For this review, take the finished solid that the model builds, in its own axes (mm). Face numbers are marked on the shaded views. A direction names the side the tool comes from. Round coordinates to 2 decimals unless told otherwise and drop trailing zeros. Order: outer loops, then holes, each group sorted by start corner. A loop starts at its lowest first (then second) coordinate and runs counter-clockwise, first axis right, second up. Notation, with made-up numbers: (12, -29) -> (28, -29) arc R4 ccw to (28, -23) -> close; hole circle Ø6 at (80.5, -19). An arc over 180 degrees is marked (long way). Answer in a Markdown table with one row per item.
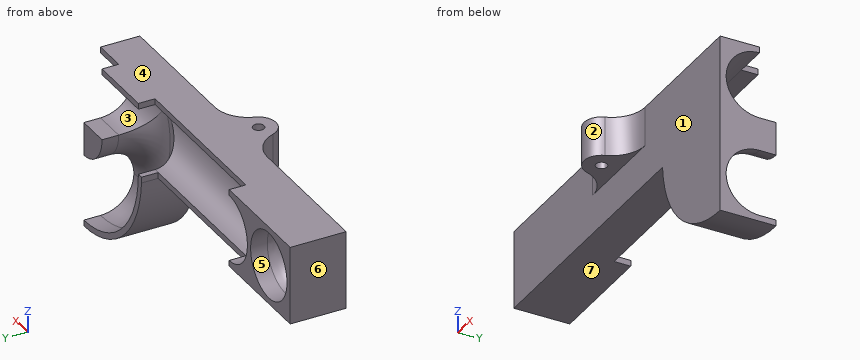
Autodesk Inventor part; units mm, degrees
ref_plane "YZ Plane" through (0, 0, 0) normal (1, 0, 0) x (0, 1, 0)
ref_plane "XZ Plane" through (0, 0, 0) normal (0, 1, 0) x (-1, 0, 0)
ref_plane "XY Plane" through (0, 0, 0) normal (0, 0, 1) x (1, 0, 0)
sketch "Esboço1" plane through (0, 0, 0) normal (0, 1, 0) x (-1, 0, 0)
  arc A0 (-102.2, -28.6) -> (-93.2, -19.6) centre (-102.2, -19.6) ccw
  arc A1 (-102.2, -46.6) -> (-75.2, -19.6) centre (-102.2, -19.6) ccw
  line L0 (-75.2, -19.6) -> (-30.2, -19.6)
  line L1 (-93.2, -19.6) -> (-102.2, -19.6)
  line L2 (-102.2, -19.6) -> (-102.2, -1.6)
  line L3 (-102.2, -1.6) -> (-93.2, -1.6)
  line L4 (-93.2, -1.6) -> (-75.2, -1.6)
  line L5 (-75.2, -1.6) -> (-30.2, -1.6)
  arc A2 (-30.2, -19.6) -> (-30.2, -1.6) centre (-30.2, -10.6) ccw
  line L6 (-102.2, -28.6) -> (-102.2, -46.6)
  arc A3 (-102.2, -48.2) -> (-73.6448, -21.2) centre (-102.2, -19.6) ccw
  arc A4 (-102.2, -27) -> (-94.975, -21.2) centre (-102.2, -19.6) ccw
  line L7 (-94.975, -21.2) -> (-102.2, -21.2)
  line L8 (-102.2, 0) -> (-93.2, 0)
  line L9 (-93.2, 0) -> (-75.2, 0)
  line L10 (-75.2, 0) -> (0, 0)
  line L11 (0, -21.2) -> (-73.6448, -21.2)
  line L12 (-73.6448, -21.2) -> (-73.6448, -19.6)
  line L13 (-102.2, -46.6) -> (-102.2, -48.2)
  line L14 (-102.2, -28.6) -> (-102.2, -27)
  line L15 (-102.2, -21.2) -> (-102.2, -19.6)
  line L16 (-102.2, -1.6) -> (-102.2, 0)
  line L17 (-94.975, -21.2) -> (-94.975, -19.6)
  line L18 (-93.2, -1.6) -> (-93.2, 0)
  line L19 (-75.2, -1.6) -> (-75.2, 0)
  line L20 (0, -21.2) -> (0, 0)
  circle A5 centre (-10.6, -10.6) radius 9
  line L21 (-30.2, -21.2) -> (-30.2, -19.6)
  line L22 (-30.2, -1.6) -> (-30.2, 0)
  line L23 (-102.2, -21.2) -> (-102.2, -27)
  point P0 (-21.2, -10.6)
  point P1 (-73.6448, -21.2)
  point P2 (-30.2, -1.6)
  point P3 (-30.2, -19.6)
  dimension "d20" = 18
  dimension "d21" = 18
  dimension "d22" = 54
  dimension "d23" = 1.6
  dimension "d30" = 1.6
  dimension "d31" = 1.6
  dimension "d32" = 1.6
  dimension "d33" = 9
  dimension "d35" = 18
  dimension "d38" = 1.6
  dimension "d44" = 1.6
  dimension "d45" = 1.6
extrude "Margem externa" add sketch "Esboço1" against normal blind 1.6 contours L14 A4 L17 L1 A0 | A0 L1 L2 L3 L4 L5 A2 L0 A1 L6 | A1 L0 L12 A3 L13 | L23 L7 A4 | L17 L7 L15 L1 | L0 L21 L11 L12 | L16 L8 L18 L3 | A2 L22 L10 L20 L11 L21 | L18 L9 L19 L4 | L5 L19 L10 L22 | A5
extrude "Proteção alta" add sketch "Esboço1" along normal blind 13.5 contours L14 A4 L17 L1 A0 | A1 L0 L12 A3 L13 | L23 L7 A4 | L17 L7 L15 L1 | A2 L22 L10 L20 L11 L21 | L18 L9 L19 L4
extrude "Proteção baixa" add sketch "Esboço1" along normal blind 9 contours L14 A4 L17 L1 A0 | A1 L0 L12 A3 L13 | L17 L7 L15 L1 | L0 L21 L11 L12 | L16 L8 L18 L3 | A2 L22 L10 L20 L11 L21 | L18 L9 L19 L4 | L5 L19 L10 L22
fillet "Arredondamento3" radius 9 7 edges at (19.6, 0, -10.6) (66.2, 0, -1.6) (52.7, 0, -19.6) (21.2, 0, -10.6) (83.1081, 0, -38.6919) (97.7, 0, -19.6) (95.836, 0, -25.964)
sketch "Esboço2" plane through (0, -1.6, 0) normal (0, -1, 0) x (1, 0, 0)
  line L0 (59.514, 0) -> (44.514, 0)
  line L1 (44.514, 0) -> (44.514, -10.6)
  line L2 (44.514, -10.6) -> (59.514, -10.6)
  line L3 (59.514, -10.6) -> (59.514, 0)
  line L4 (0, 0) -> (0, -21.2)
  point P0 (52.014, -10.6)
  point P1 (0, -10.6)
  point P2 (52.014, 0)
  dimension "d47" = 52.014
  dimension "d48" = 15
extrude "Extrusão5" add sketch "Esboço2" along normal blind 9.4
sketch "Esboço3" plane through (59.514, -1.6, -10.6) normal (0, 0, -1) x (-1, 0, 0)
  circle A0 centre (7.5, -4.7) radius 1.5
  line L0 (15, -9.4) -> (0, -9.4)
  line L1 (15, 0) -> (15, -9.4)
  line L2 (59.514, 0) -> (-14.1308, 0)
  line L3 (12.2, 0) -> (15, 0)
  line L4 (15, 0) -> (15, -9.4)
  line L5 (15.1598, -9.4) -> (0, -9.4)
  line L6 (0, -9.4) -> (0, 0)
  line L7 (0, 0) -> (2.8, 0)
  circle A1 centre (7.5, -4.7) radius 4.7
  line L8 (12.2, 0) -> (12.2, -4.7)
  line L9 (2.8, 0) -> (2.8, -4.7)
  point P0 (59.514, 1.6)
  point P1 (7.5, -9.4)
  point P2 (15, -4.7)
  point P3 (9, -4.7)
  point P4 (6, -4.7)
  point P5 (7.5, -9.4)
  dimension "d51" = 3
  dimension "d54" = 3.2
extrude "Extrusão6" cut sketch "Esboço3" against normal through all contours A0 | L0 A1 L8 L2 L1 | L0 L6 L2 L9 A1
fillet "Arredondamento4" radius 9 2 edges at (56.714, -1.6, -5.3) (47.314, -1.6, -5.3)
equation "\"d20\" = Esfera"
equation "\"d21\" = Esfera"
equation "\"d23\" = Margem"
equation "\"d30\" = Margem"
equation "\"d31\" = Margem"
equation "\"d28\" = Margem"
equation "\"d24\" = 0.75 * Esfera"
equation "\"Esfera\" = 18"
equation "\"Margem\" = 1.6"
equation "\"Furo\" = 3"
properties part number "Trilho 5 min" material "Plástico PET"
Q1. To check wall thickness, follow probe 1 along Z at (x, y) = (10.6, 11.8); probe 2 along X at (y, z) = (10.5, -10); probe 3 along Y at (x, z) = (92.5, -35.5). State the ranges of each line that lie inside material, in increasing order.
Answer key:
| item | result |
|---|---|
| probe 1 | z = -21.2 to -19.6, -1.6 to 0 |
| probe 2 | x = 0 to 1.62, 19.58 to 21.22 |
| probe 3 | y = -1.6 to 0.02 |
Q2. Clearance check with flat-ended pins moving along their axes: pin 1 Ø3 at (y, z) = (3, -39.5) entering from -X; pin 2 Ø14.5 at (x, z) = (10.6, -10.6) entering from -Y; pin 3 Ø3.5 at (x, y) = (96.5, 12) entering from +Z; pin 4 Ø3.5 at (x, y) = (48.5, 12) entering from -Z. State where each tip first meets the part, or that it passes through.
Answer key:
| item | result |
|---|---|
| pin 1 | stops at x = 80.3 |
| pin 2 | stops at y = -1.6 |
| pin 3 | stops at z = -19.6 |
| pin 4 | passes through |
Q3. Take a section at B-B, the plane y = 2.25. Give the number of separate pieces and of enclosed holes in the cut face, then the cut area to 3 significant figures.
Answer key:
| item | result |
|---|---|
| separate pieces | 2 |
| enclosed holes | 1 |
| area | 1,370 mm^2 |
Q4. Take a section at A-A, the plane y = -6.3. Write out the cut boundary in (x, z), then the cut area to 3 significant figures.
Answer key:
| item | result |
|---|---|
| outline | (46.91, -10.6) -> (50.51, -10.6) -> (50.51, 0) -> (46.91, 0) -> close; (53.51, -10.6) -> (57.12, -10.6) -> (57.12, 0) -> (53.51, 0) -> close |
| area | 76.3 mm^2 |
Q5. Tool access review of the marked faces 1, 2 and 3: name each direction out of +Z, -Z, +X, -X, +Y, -Y from which nothing blocks a thin tool from reaching the whole face with its end or side.
Answer key:
| item | result |
|---|---|
| face 1 | -Z, -Y |
| face 2 | +Z, -Z, -Y |
| face 3 | +X, +Y |
Q6. The part is to be moulded in two halves that separate along Z. For the marked faces 4, 5, 6 and 7, say which applies: +Z half, -Z half, draft (parallel to the pull), parting line (faces both ways), or undercut.
Answer key:
| item | result |
|---|---|
| face 4 | +Z half |
| face 5 | undercut |
| face 6 | draft |
| face 7 | -Z half |
